The model under review builds one solid part; all positions refer to its coordinate system, in mm. A direction names the side the tool comes from. Round coordinates to 2 decimals unless told otherwise and drop trailing zeros. Loops run counter-clockwise (first coordinate to the right, second up) from the corner with the lowest first, then second, coordinate; pieces in that order, holes last. Notation, with made-up numbers: (53.25, -37.75) -> (107.25, -37.75) arc R5 ccw to (107.25, -31.75) -> close; hole circle Ø2 at (24.5, -5.75). An arc over 180 degrees is marked (long way). Return JSON: item names as keys, results as strings. Group by question number.
Autodesk Inventor part; units mm, degrees
ref_plane "Work Plane2" through (0, 21.12, 0) normal (0, 1, 0) x (-1, 0, 0)
ref_plane "YZ Plane" through (0, 0, 0) normal (1, 0, 0) x (0, 1, 0)
ref_plane "XY Plane" through (0, 0, 0) normal (0, 0, 1) x (1, 0, 0)
sketch "Sketch1" plane through (0, 0, 0) normal (0, 0, 1) x (1, 0, 0)
  circle A0 centre (0, 0) radius 19.12
extrude "Extrusion1" add sketch "Sketch1" against normal blind 34.12
fillet "Fillet1" radius 1 1 edges at (-19.12, 0, -34.12)
sketch "Sketch2" plane through (0, 0, 0) normal (0, 0, 1) x (1, 0, 0)
  circle A0 centre (0, 0) radius 19.12
  circle A1 centre (0, 0) radius 19.37
extrude "Extrusion2" add sketch "Sketch2" against normal blind 2
sketch "Sketch3" plane through (0, 0, 0) normal (0, 0, 1) x (1, 0, 0)
  circle A0 centre (0, 0) radius 19.37
  circle A1 centre (0, 0) radius 10
extrude "Extrusion3" add sketch "Sketch3" along normal blind 5 contours A1
sketch "Sketch4" plane through (0, 0, 5) normal (0, 0, 1) x (1, 0, 0)
  circle A0 centre (0, 0) radius 10
  circle A1 centre (0, 0) radius 7.14
extrude "Extrusion4" cut sketch "Sketch4" against normal blind 5 contours A1
sketch "Sketch5" plane through (0, 0, 0) normal (0, 0, 1) x (1, 0, 0)
  circle A0 centre (0, 0) radius 7.14
  circle A1 centre (0, 0) radius 3.83
extrude "Extrusion5" add sketch "Sketch5" along normal blind 4 contours A1
sketch "Sketch6" plane through (0, 0, 4) normal (0, 0, 1) x (1, 0, 0)
  circle A0 centre (0, 0) radius 3.83
  circle A1 centre (0, 0) radius 3
extrude "Extrusion6" add sketch "Sketch6" along normal blind 13.4 contours A1
sketch "Sketch7" plane through (0, 0, 17.4) normal (0, 0, 1) x (1, 0, 0)
  circle A0 centre (0, 0) radius 3
  line L0 (0, 2.8) -> (1.077033, 2.8)
  line L1 (0, 2.8) -> (-1.077033, 2.8)
  arc A1 (1.077033, 2.8) -> (0, 3) centre (0, 0) ccw
  arc A2 (0, 3) -> (-1.077033, 2.8) centre (0, 0) ccw
extrude "Extrusion7" cut sketch "Sketch7" against normal blind 10 contours L0 L1 A0 picked at (-0.601378, 2.836851)
fillet "Fillet2" radius 0.3 2 edges at (-10, 0, 5) (-10, 0, 0)
chamfer "Chamfer1" distance 0.3 angle 45 1 edges at (-7.14, 0, 5)
sketch "Sketch8" plane through (0, 0, 0) normal (0, 0, 1) x (1, 0, 0)
  circle A0 centre (0, 0) radius 3.83
  circle A1 centre (0, 0) radius 7.14
  circle A2 centre (0, 0) radius 7.1
sketch "Sketch8 outline for Extrusion8" plane through (0, 0, 0) normal (0, 0, 1) x (1, 0, 0)
  circle A0 centre (0, 0) radius 7.1
  circle A1 centre (0, 0) radius 3.83
extrude "Extrusion8" add sketch "Sketch8 outline for Extrusion8" along normal blind 3.8
sketch "Sketch9" plane through (0, 0, 0) normal (0, 0, 1) x (1, 0, 0)
  circle A0 centre (0, 0) radius 19.37
  circle A1 centre (0, 14.835) radius 1.25
  circle A2 centre (-12.847487, -7.4175) radius 1.25
  circle A3 centre (12.847487, -7.4175) radius 1.25
  circle A4 centre (6.2, 14.835) radius 1.25
  circle A5 centre (-15.947487, -2.048142) radius 1.25
  circle A6 centre (9.747487, -12.786858) radius 1.25
  dimension "d32" = 360
  dimension "d38" = 360
extrude "Extrusion9" cut sketch "Sketch9" against normal blind 5 contours A1 | A2 | A3 | A4 | A5 | A6
thread "Thread1"
thread "Thread2"
thread "Thread3"
thread "Thread4"
thread "Thread5"
thread "Thread6"
chamfer "Chamfer2" distance 0.3 angle 45 6 edges at (-1.25, 14.835, 0) (4.95, 14.835, 0) (11.5975, -7.4175, 0) (8.4975, -12.7869, 0) (-14.0975, -7.4175, 0) (-17.1975, -2.0481, 0)
ref_plane "Work Plane2" through (0, 21.12, 0) normal (0, 1, 0) x (-1, 0, 0)
ref_plane "Work Plane1" through (0, 19.12, 0) normal (0, 1, 0) x (-1, 0, 0)
sketch "Sketch10" plane through (0, 21.12, 0) normal (0, 1, 0) x (-1, 0, 0)
  line L0 (18.12, -34.12) -> (-18.12, -34.12)
  line L1 (-19.12, -33.12) -> (19.12, -33.12)
  line L2 (0, -33.12) -> (0, -26.12)
  circle A0 centre (0, -26.12) radius 5
  circle A1 centre (0, -26.12) radius 2.5
  point P0 (0, 0)
extrude "Extrusion10" add sketch "Sketch10" against normal blind 5
properties part number "Rotary Encoder"
1. Tool access review of faces 4 (the face through (0, 15, -5)), 5 (the face through (0, 2.8, 12)): name each direction out of +Z, -Z, +X, -X, +Y, -Y from which nothing blocks a thin tool from reaching the whole face with its end or side.
2. We need section B-B, the plane z = -9.5. Write out the cut boundary in (x, y), then the cut area to 3 significant figures.
3. We need section C-C, the plane z = 10.5. Write out the cut boundary in (x, y).
4. Draft analysis for pull direction X (two halves, no side actions). For faces 1 (the face through (-2.17, 9.76, 2.47)), 2 (the face through (-2, 21.12, -28)), 3 (the face through (6, 15, -5)), state which applies: pulls with the +X half, pulls with the -X half, needs draft (parallel to the pull), parting line crosses it, or undercut.
5. Wall thickness on line 1 (Y direction, x = 0, z = -3) (3 decimals); line 2 (Z direction, x = 8.5, y = -15.5); line 3 (X direction, y = 19.85, z = -26.12): over which ranges is each line inside the solid? List them lowest first.
6. For P1, Ø2, axis at x = -15.95, y = -2.05, coming from the +Z side; P2, Ø2, axis at x = -1, z = -23, coming from the -Y side; P3, Ø1, axis at y = 10, z = -19.5, coming from the +X side, all flat-tipped, find the tip position at first contact; note any pin that passes through.
7. We need section A-A, the plane z = -26.12. Write out the cut boundary in (x, y).
Check sheet entries:
{
 "1": {"face 4": "+Z", "face 5": "+Z, +X, -X, +Y"},
 "2": {"outline": "circle Ø38.24 at (0, 0)", "area": "1,150 mm²"},
 "3": {"outline": "(-1.08, 2.8) arc R3 ccw (long way) to (1.08, 2.8) -> close"},
 "4": {"face 1": "parting line crosses it", "face 2": "needs draft", "face 3": "undercut"},
 "5": {"line 1": "y = -19.12 to 13.585, 16.085 to 19.12", "line 2": "z = -34.12 to 0", "line 3": "x = -5 to -2.5, 2.5 to 5"},
 "6": {"P1": "stops at z = -5", "P2": "stops at y = -19.12", "P3": "stops at x = 16.59"},
 "7": {"outline": "(-5, 18.45) arc R19.12 ccw (long way) to (5, 18.45) -> (5, 21.12) -> (2.5, 21.12) -> (2.5, 18.96) arc R19.12 ccw to (-2.5, 18.96) -> (-2.5, 21.12) -> (-5, 21.12) -> close"}
}
